Geometry check sheet. Reference: the model listing, model coordinates, mm. Face numbers are marked on the shaded views. A direction names the side the tool comes from. Coordinates: 2 decimals unless noted, no trailing zeros. Write each loop counter-clockwise with the first axis right and the second up, starting at its lowest first coordinate (ties: lowest second). Pieces come first, ordered by that corner, then holes. Notation, with made-up numbers: (71, 35.5) -> (80, 35.5) arc R27 ccw to (80, 64.5) -> close; hole circle Ø4 at (2.25, 26.5). An arc over 180 degrees is marked (long way). Use a Markdown table: item, result.
```python
from build123d import *

# Parameters (mm, degrees)
F1_DEPTH = 15


with BuildPart() as f1:
    # F0 (on Top) → F1 (new body, symmetric)
    with BuildSketch(Plane.XY):
        with BuildLine():
            ThreePointArc((12.562231, -10.927619), (-15.152019, -6.902088), (0, 16.65))
            Line((0, 16.65), (14, 16.65))
            ThreePointArc((14, 16.65), (15.5, 16.01501), (16.088171, 14.496041))
            Line((16.088171, 14.496041), (18.793797, 14.496041))
            add(Edge.make_bspline(
                [(10.105219, 26.496041), (18.016234, 24.516107), (20.053543, 19.857231), (18.793797, 14.496041)],
                knots=[0, 0, 0, 0, 14.815242, 14.815242, 14.815242, 14.815242], degree=3))
            add(Edge.make_bspline(
                [(10.105219, 26.496041), (12.580878, 24.072407), (15.021241, 21.072751), (9, 18.5)],
                knots=[0, 0, 0, 0, 8.072061, 8.072061, 8.072061, 8.072061], degree=3))
            Line((9, 18.5), (0, 18.5))
            ThreePointArc((0, 18.5), (-17.775458, 5.126704), (-9.851839, -15.658585))
            ThreePointArc((-9.851839, -15.658585), (-9.609354, -15.789858), (-9.381345, -15.944917))
            ThreePointArc((-9.381345, -15.944917), (-8.310595, -17.863662), (-9, -19.95))
            Line((-9, -19.95), (9, -19.95))
            ThreePointArc((9, -19.95), (10.869586, -15.862711), (14.907399, -13.888538))
            Line((14.907399, -13.888538), (17.907399, -13.888538))
            ThreePointArc((17.907399, -13.888538), (20.110659, -13.224193), (21.440358, -11.345999))
            Line((21.440358, -11.345999), (22.189979, -8.788404))
            ThreePointArc((22.189979, -8.788404), (20.902351, -7.06921), (19.614723, -8.788404))
            ThreePointArc((19.614723, -8.788404), (19.086815, -9.963811), (17.857542, -10.35002))
            Line((17.857542, -10.35002), (14.042224, -10.35002))
            ThreePointArc((14.042224, -10.35002), (13.231128, -10.456638), (12.562231, -10.927619))
        make_face()
        with BuildLine():
            ThreePointArc((-9.381345, -15.944917), (-9.609354, -15.789858), (-9.851839, -15.658585))
            ThreePointArc((-9.851839, -15.658585), (-9.617657, -15.803502), (-9.381345, -15.944917))
        make_face()
    extrude(amount=F1_DEPTH, both=True)


solid = f1.part
```
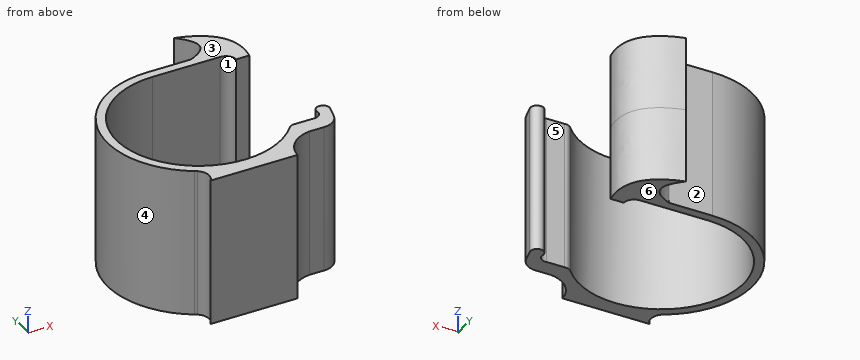
Item 1: Section check B-B on y = 0. Record the boundary of the cut face in (x, z).
Answer block:
| item | result |
|---|---|
| outline | (-18.5, -15) -> (-16.65, -15) -> (-16.65, 15) -> (-18.5, 15) -> close |
Item 2: Tool access check on the marked faces 5 and 6. Record the directions out of +Z, -Z, +X, -X, +Y, -Y that give a thin tool (end or side, any length) a straight path to the whole face; none if there is none.
Answer block:
| item | result |
|---|---|
| face 5 | +Z, -Z |
| face 6 | -Z, +X, -X, +Y, -Y |
Item 3: Mould release check, pull along Y, two halves, no side actions. Record for the marked faces 1, 2, 3 and 4: +Y half, -Y half, draft (parallel to the pull), parting line (faces both ways), or undercut.
Answer block:
| item | result |
|---|---|
| face 1 | undercut |
| face 2 | +Y half |
| face 3 | draft |
| face 4 | parting line |
Item 4: Section check C-C on x = 7. Record the boundary of the cut face in (y, z).
Answer block:
| item | result |
|---|---|
| outline | (-19.95, -15) -> (-15.11, -15) -> (-15.11, 15) -> (-19.95, 15) -> close; (16.65, -15) -> (18.5, -15) -> (18.5, 15) -> (16.65, 15) -> close |
Item 5: Depth check by flat-ended pin: P1, Ø4, axis at x = -7, z = -2.5, coming from the +Y side; P2, Ø3, axis at x = 11.5, y = -11.5, coming from the +Z side; P3, Ø4.5, axis at x = 3.5, z = -2, coming from the +Y side; P4, Ø10, axis at y = 9, z = -2, coming from the +X side. Enter the tip coordinate at first touch or a pass-through.
Answer block:
| item | result |
|---|---|
| P1 | stops at y = 17.81 |
| P2 | stops at z = 15 |
| P3 | stops at y = 18.5 |
| P4 | stops at x = -9.01 |
Item 6: Thickness scan on L1, parallel to X at y = 0, z = -3; L2, parallel to Y at x = -3, z = 5; L3, parallel to X at y = -11, z = -2. Record the ranges inside material, lowest first. Write a range as [from, to].
Answer block:
| item | result |
|---|---|
| L1 | x = [-18.5, -16.65] |
| L2 | y = [-19.95, -16.38], [16.38, 18.26] |
| L3 | x = [-14.87, -12.5], [12.5, 21.54] |
Item 7: Section check A-A on x = 2.5. Record the boundary of the cut face in (y, z), then the cut area to 3 significant figures.
Answer block:
| item | result |
|---|---|
| outline | (-19.95, -15) -> (-16.46, -15) -> (-16.46, 15) -> (-19.95, 15) -> close; (16.65, -15) -> (18.5, -15) -> (18.5, 15) -> (16.65, 15) -> close |
| area | 160 mm^2 |
